```python
from build123d import *

# Parameters (mm, degrees)
F0_W     = 0.8717233978
F0_H     = 0.6
F1_DEPTH = 2.5
F2_DEPTH = 0.6
F4_SIZE  = 0.59999
F5_R     = 0.7
F6_R     = 1
F7_R     = 0.15


# Not quite as in the source:
# - a fillet or chamfer is up to 0.001 mm smaller than in the source, because OpenCascade refuses the exact size


with BuildPart() as f1:
    # F0 (on Front) → F1 (new body)
    with BuildSketch(Plane.XZ):
        Polygon((0, 1), (0, 0), (3, 0), (2, 1), (0.7, 1), align=None)
        Polygon((2.7075850967, 9.087372576), (1.8358616989, 9.087372576), (3.5531366706, 7.8849236956), (1.8358616989, 6.7266071015), (3.5531366706, 5.5241582211), (1.8358616989, 4.365841627), (3.5531366706, 3.1633927466), (1.8358616989, 2.0050761525), (2.7, 1.4), (3.5717233978, 1.4), (2.7185867272, 1.9973727279), (4.4358616989, 3.155689322), (2.7185867272, 4.3581382024), (4.4358616989, 5.5164547965), (2.7185867272, 6.7189036769), (4.4358616989, 7.877220271), align=None)
        with Locations((3.1358616989, 1.1)):
            Rectangle(F0_W, F0_H)
        Polygon((0, 9), (0, 1), (0.7, 1), (0.7, 9.087372576), (1.8358616989, 9.087372576), (2.7075850967, 9.087372576), (4, 9.087372576), (4, 10), (0, 10), align=None)
    extrude(amount=F1_DEPTH)

    # F0 (on Front) → F2 (join)
    with BuildSketch(Plane.XZ):
        Polygon((0, 1), (0, 0), (3, 0), (2, 1), (0.7, 1), align=None)
    extrude(amount=-F2_DEPTH)

    # F3: F1 across face


with BuildPart() as f1_1:
    add(f1.part)
    add(f1.part.mirror(Plane(origin=(0, -1.213671875, 4.89453125), x_dir=(0, -1, 0), z_dir=(-1, 0, 0))))

    # F4 (size 0.6 in the source; OpenCascade refuses exactly that, so slightly less here)
    f4_edges = [f1_1.edges().sort_by_distance(p)[0] for p in [
        (0, 0.6, 1),
    ]]
    chamfer(f4_edges, length=F4_SIZE)

    # F5
    f5_edges = [f1_1.edges().sort_by_distance(p)[0] for p in [
        (0.7, -1.25, 9.087373),
        (-0.7, -1.25, 9.087373),
        (1.835862, -1.25, 9.087373),
        (-1.835862, -1.25, 9.087373),
    ]]
    fillet(f5_edges, radius=F5_R)

    # F6
    f6_edges = [f1_1.edges().sort_by_distance(p)[0] for p in [
        (0.7, -1.25, 1),
        (-0.7, -1.25, 1),
    ]]
    fillet(f6_edges, radius=F6_R)

    # F7
    f7_edges = [f1_1.edges().sort_by_distance(p)[0] for p in [
        (2.707585, -1.25, 9.087373),
        (-2.707585, -1.25, 9.087373),
    ]]
    fillet(f7_edges, radius=F7_R)


solid = f1_1.part
```
Input: part model. Units: mm. Frame: model coordinates. A direction names the side the tool comes from. Give positions to 0.01 mm unless a question says otherwise; leave off trailing zeros. Loops run counter-clockwise (first coordinate to the right, second up) from the corner with the lowest first, then second, coordinate; pieces in that order, holes last.
1) Mould query, pull axis X, two halves, no side actions, for faces 5 (the flat face through (3.59, -1.23, 3.75)), 6 (the flat face through (-3.57, -1.23, 2.57)), 7 (the flat face through (0, -2.5, 5)), 8 (the flat face through (2.682, -1.232, 3.773)). Classes: released by +X, released by -X, zero draft, split by the parting line, or undercut.
A:
face 5: released by +X
face 6: released by -X
face 7: zero draft
face 8: undercut
2) Contact query for flat-ended pins moving along their axis: pin 1 (0.5 mm diameter, centred on y = -0.5, z = 1, fed in from +X); pin 2 (1 mm diameter, centred on x = 3, z = 4.5, fed in from +Y); pin 3 (5 mm diameter, centred on x = 1.5, z = 2.5, fed in from -Y); pin 4 (0.7 mm diameter, centred on y = -0.5, z = 9.5, fed in from +X). Output: stop coordinate, or through.
A:
pin 1: stops at x = 3.57
pin 2: stops at y = 0
pin 3: stops at y = -2.5
pin 4: stops at x = 4
3) Section query C-C on z = 7.75. Return the cut outline in (x, y), and give its area (3 significant figures).
A:
outline: (-4.25, -2.5) - (-3.35, -2.5) - (-3.35, 0) - (-4.25, 0) - close; (-0.7, -2.5) - (0.7, -2.5) - (0.7, 0) - (-0.7, 0) - close; (3.35, -2.5) - (4.25, -2.5) - (4.25, 0) - (3.35, 0) - close
area: 7.97 mm2
4) Section query B-B on z = 4. Return the cut outline in (x, y), and give its area (3 significant figures).
A:
outline: (-3.23, -2.5) - (-2.36, -2.5) - (-2.36, 0) - (-3.23, 0) - close; (-0.7, -2.5) - (0.7, -2.5) - (0.7, 0) - (-0.7, 0) - close; (2.36, -2.5) - (3.23, -2.5) - (3.23, 0) - (2.36, 0) - close
area: 7.86 mm2
5) Line query: L1, parallel to X at y = -1.3, z = 3; L2, parallel to X at y = -1.65, z = 5.75; L3, parallel to Z at x = 3.75, y = -1.55. Output: solid intervals per line, ascending.
A:
L1: x = -4.21 to -3.31, -0.7 to 0.7, 3.31 to 4.21
L2: x = -4.1 to -3.23, -0.7 to 0.7, 3.23 to 4.1
L3: z = 2.69 to 3.64, 5.05 to 6, 7.41 to 8.36, 9.09 to 10
6) Reachability of faces 1 (the flat face through (-3.6, -1.2, 9.087)), 2 (the flat face through (3, -1, 0.8)), 3 (the flat face through (-2.26, -1.23, 1.71)), 4 (the flat face through (-4, -1.2, 9.5)) from +Z, -Z, +X, -X, +Y, -Y: full face, straight path, thin tool, end or side. Return the list, or none.
A:
face 1: -X, +Y, -Y
face 2: +X, +Y, -Y
face 3: +Y, -Y
face 4: +Z, -X, +Y, -Y
